The listing builds one solid part. Answer for the finished solid, in the listing's coordinates (mm). Face numbers are marked on the shaded views. A direction names the side the tool comes from. Round coordinates to 2 decimals unless told otherwise and drop trailing zeros. Write each loop counter-clockwise with the first axis right and the second up, starting at its lowest first coordinate (ties: lowest second). Pieces come first, ordered by that corner, then holes. Notation, with made-up numbers: M 86.5,29 L 115.5,29 A30 cw 115.5,56 Z; hole C 83.5,16.5 d3. An arc over 180 degrees is marked long. One line per item, written item: value. Start each with the question number.
(1) Section A-A (z = 1.4) is taken. State how many separate pieces and enclosed holes the cut face has, plus the area to 3 significant figures.
(2) For the marked faces 4, 5 and 6, determine the directions among +Z, -Z, +X, -X, +Y, -Y from which every point of the face is accessible in a straight line to the end or side of a thin tool.
(3) Section B-B (y = 9) is taken. Determine the outline of the cut face in (x, z), plus the area to 3 significant figures.
(4) For a pull along Y with two mould halves and no side action, classify the marked faces 1, 2 and 3 as released by +Y, released by -Y, zero draft, split by the parting line, or undercut.
(5) Section C-C (x = -2) is taken. Determine the outline of the cut face in (y, z).
(6) Consider probe 1 along X at (y, z) = (9, 1.6); probe 2 along Y at (x, z) = (-0.5, 0.6); probe 3 along Y at (x, z) = (2.75, 0.2). Determine where each line is inside the solid, lowest interval first.
(7) Given P1, Ø0.5, axis at y = 8.5, z = 1, coming from the -X side; P2, Ø1.8, axis at x = 0, y = 14.86, coming from the +Z side; P3, Ø0.7, axis at y = 14, z = 0.5, coming from the +X side, each flat-ended and moving along its own axis, determine where each tip first touches the part or whether it passes through.
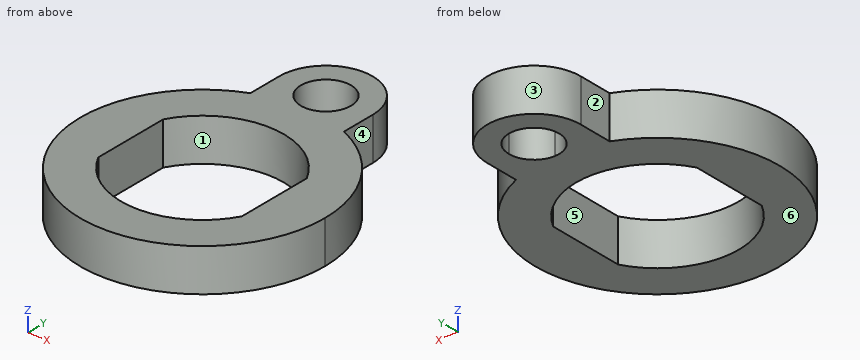
```python
from build123d import *

# Parameters (mm, degrees)
F1_DEPTH = 1.651


with BuildPart() as f1:
    # F0 (on Top) → F1 (new body)
    with BuildSketch(Plane.XY):
        with BuildLine():
            ThreePointArc((1.8213407221, 13.5264450688), (0.9284865025, 13.7970918303), (2e-09, 13.8884764319))
            ThreePointArc((2e-09, 13.8884764319), (-0.9284865005, 13.7970918307), (-1.8213407221, 13.5264450688))
            ThreePointArc((-1.8213407221, 13.5264450688), (-2.6464382726, 5.1664599565), (4.7625, 9.1259764319))
            ThreePointArc((4.7625, 9.1259764319), (3.9595164755, 11.7724147045), (1.8213407221, 13.5264450688))
        make_face()
        with BuildLine():
            ThreePointArc((-2.794, 10.634017877), (0, 12.3009764319), (2.794, 10.634017877))
            Line((2.794, 10.634017877), (2.794, 7.6179349869))
            ThreePointArc((2.794, 7.6179349869), (0, 5.9509764319), (-2.794, 7.6179349869))
            Line((-2.794, 7.6179349869), (-2.794, 10.634017877))
        make_face(mode=Mode.SUBTRACT)
        with BuildLine():
            ThreePointArc((-1.8213407221, 13.5264450688), (-0.9284865005, 13.7970918307), (2e-09, 13.8884764319))
            ThreePointArc((2e-09, 13.8884764319), (0.9284865025, 13.7970918303), (1.8213407221, 13.5264450688))
            Line((1.8213407221, 13.5264450688), (1.8213407221, 14.8630785568))
            ThreePointArc((1.8213407221, 14.8630785568), (0, 16.6844192788), (-1.8213407221, 14.8630785568))
            Line((-1.8213407221, 14.8630785568), (-1.8213407221, 13.5264450688))
        make_face()
        with BuildLine():
            ThreePointArc((2e-09, 13.8884764319), (-0.6891477722, 15.5522263275), (0.9746021248, 14.8630785568))
            ThreePointArc((0.9746021248, 14.8630785568), (0.6891477722, 14.173930786), (2e-09, 13.8884764319))
        make_face(mode=Mode.SUBTRACT)
    extrude(amount=F1_DEPTH)


solid = f1.part
```
Recorded:
1. separate pieces: 1
1. enclosed holes: 2
1. area: 47.3 mm2
2. face 4: +Z, -Z, +X, +Y
2. face 5: +Z, -Z
2. face 6: -Z, +X, -X, +Y, -Y
3. outline: M -4.76,0 L -2.79,0 L -2.79,1.65 L -4.76,1.65 Z; M 2.79,0 L 4.76,0 L 4.76,1.65 L 2.79,1.65 Z
3. area: 6.49 mm2
4. face 1: undercut
4. face 2: zero draft
4. face 3: released by +Y
5. outline: M 4.8,0 L 6.66,0 L 6.66,1.65 L 4.8,1.65 Z; M 11.59,0 L 13.45,0 L 13.45,1.65 L 11.59,1.65 Z
6. probe 1: x = -4.76 to -2.79, 2.79 to 4.76
6. probe 2: y = 4.39 to 5.99, 12.26 to 14.03, 15.7 to 16.61
6. probe 3: y = 5.24 to 7.54, 10.71 to 13.01
7. P1: stops at x = -4.75
7. P2: passes through
7. P3: stops at x = 1.82
